Part model, mm, in its own coordinate system. A direction names the side the tool comes from. Coordinates: 2 decimals unless noted, no trailing zeros. Loops run counter-clockwise (first coordinate to the right, second up) from the corner with the lowest first, then second, coordinate; pieces in that order, holes last. Notation, with made-up numbers: (85, 34) - (125, 34) arc R16 ccw to (125, 41) - close; hole circle Ø8 at (21, -36). An arc over 180 degrees is marked (long way). Use a Markdown table: item, result. Add a question column.
1. 3-axis set-ups, long thin cutter, end or side, ignore diameter. For faces 1 (the flat face through (13, -15, 10.365)), 2 (the cylindrical face through (7.269, -8.265, 11.351)), 3 (the flat face through (-2.959, -15, -2)): which of +Z, -Z, +X, -X, +Y, -Y reach the whole face in a straight line?
2. Drop a flat-ended pin along its axis: pin 1 (4.5 mm diameter, centred on x = 7.04, y = -20, fed in from -Z). Give the stop position or say it passes through.
3. Pull direction Z, two halves, no side cores. Call faces 4 (the cylindrical face through (18.331, -13.817, 11.351)), 5 (the flat face through (-0.959, -15, -3)), 6 (the flat face through (2.066, -14.79, -21.763)): pulls with the +Z half, pulls with the -Z half, needs draft (parallel to the pull), parting line crosses it, or undercut.
4. Band-saw the part on C-C, the plane y = -24.75. Give the cut face in (x, z).
5. Band-saw the part on D-D, the plane z = -16. Give the cut face in (x, y).
6. Band-saw the part on B-B, the plane x = 16.5. Give the cut face in (y, z), plus the area to 3 significant figures.
7. Band-saw the part on A-A, the plane y = -10. Give the cut face in (x, z).
8. Wall check: probe 1 along Z at (x, y) = (17, -23); probe 2 along X at (y, z) = (-4.5, -12); probe 3 along Z at (x, y) = (3.25, -18.25). Give the ranges that are in metal, low to high. Write a range as [from, to].
from build123d import *

# Parameters (mm, degrees)
F1_DEPTH = 30
F3_D     = 3.5
F3_DEPTH = 5


with BuildPart() as f1:
    # F0 (on Front) → F1 (new body)
    with BuildSketch(Plane.XZ):
        Polygon((27.040993, 12.364779), (-2.959007, 12.364779), (-2.959007, -17.635221), (7.234091, -26.008121), (8.50357, -24.462669), (-0.959007, -16.689839), (-0.959007, 10.364779), (27.040993, 10.364779), align=None)
    extrude(amount=F1_DEPTH)

    # F3
    with Locations(Plane.XY.offset(12.364779)):
        with Locations((7.040993, -10), (17.040993, -15), (7.040993, -20)):
            Hole(F3_D / 2, depth=F3_DEPTH)


solid = f1.part
Geometry check:
| question | item | result |
|---|---|---|
| 1 | face 1 | +X, +Y, -Y |
| 1 | face 2 | +Z |
| 1 | face 3 | +Z, -Z, -X, +Y, -Y |
| 2 | pin 1 | stops at z = -26.01 |
| 3 | face 4 | needs draft |
| 3 | face 5 | undercut |
| 3 | face 6 | pulls with the -Z half |
| 4 | outline | (-2.96, -17.64) - (7.23, -26.01) - (8.5, -24.46) - (-0.96, -16.69) - (-0.96, 10.36) - (27.04, 10.36) - (27.04, 12.36) - (-2.96, 12.36) - close |
| 5 | outline | (-2.96, -30) - (-0.96, -30) - (-0.96, 0) - (-2.96, 0) - close |
| 6 | outline | (-30, 10.36) - (-16.66, 10.36) - (-16.66, 12.36) - (-30, 12.36) - close; (-13.34, 10.36) - (0, 10.36) - (0, 12.36) - (-13.34, 12.36) - close |
| 6 | area | 53.3 mm^2 |
| 7 | outline | (-2.96, -17.64) - (7.23, -26.01) - (8.5, -24.46) - (-0.96, -16.69) - (-0.96, 10.36) - (5.29, 10.36) - (5.29, 12.36) - (-2.96, 12.36) - close; (8.79, 10.36) - (27.04, 10.36) - (27.04, 12.36) - (8.79, 12.36) - close |
| 8 | probe 1 | z = [10.36, 12.36] |
| 8 | probe 2 | x = [-2.96, -0.96] |
| 8 | probe 3 | z = [-22.74, -20.15], [10.36, 12.36] |
